Verification items for the finished model (mm, model axes). A direction names the side the tool comes from. Coordinates: 2 decimals unless noted, no trailing zeros. Write each loop counter-clockwise with the first axis right and the second up, starting at its lowest first coordinate (ties: lowest second). Pieces come first, ordered by that corner, then holes. Notation, with made-up numbers: M 72.25,24.5 L 126.25,24.5 A15 cw 126.25,40.5 Z; hole C -17,-39 d6. An arc over 180 degrees is marked long. One line per item, written item: value.
```python
from build123d import *

# Parameters (mm, degrees)
ESQUISSE1_R        = 20
ESQUISSE1_R_2      = 15
ESQUISSE1_R_3      = 6
BOSS_EXTRU_1_DEPTH = 1
ESQUISSE1_3_R      = 15
ESQUISSE1_3_R_2    = 6
BOSS_EXTRU_2_DEPTH = 12
ESQUISSE2_R        = 20
ESQUISSE2_R_2      = 15
ESQUISSE2_R_3      = 6
BOSS_EXTRU_4_DEPTH = 1


with BuildPart() as part:
    # Esquisse1 → Boss.-Extru.1 (new body)
    with BuildSketch(Plane(origin=(0, 0, 0), x_dir=(1, 0, 0), z_dir=(0, 1, 0))):
        with Locations(Location((0, 0, 0), (0, 0, 270))):
            Circle(ESQUISSE1_R)
        Circle(ESQUISSE1_R_2, mode=Mode.SUBTRACT)
        Circle(ESQUISSE1_R_2)
        with Locations(Location((0, 0, 0), (0, 0, 270))):
            Circle(ESQUISSE1_R_3, mode=Mode.SUBTRACT)
    extrude(amount=-BOSS_EXTRU_1_DEPTH)

    # Esquisse1_3 → Boss.-Extru.2 (add)
    with BuildSketch(Plane(origin=(0, 0, 0), x_dir=(1, 0, 0), z_dir=(0, 1, 0))):
        with Locations(Location((0, 0, 0), (0, 0, 270))):
            Circle(ESQUISSE1_3_R)
        with Locations(Location((0, 0, 0), (0, 0, 270))):
            Circle(ESQUISSE1_3_R_2, mode=Mode.SUBTRACT)
    extrude(amount=BOSS_EXTRU_2_DEPTH)

    # Esquisse2 → Boss.-Extru.4 (add)
    with BuildSketch(Plane(origin=(0, 12, 0), x_dir=(1, 0, 0), z_dir=(0, 1, 0))):
        with Locations(Location((0, 0, 0), (0, 0, 270))):
            Circle(ESQUISSE2_R)
        with Locations(Location((0, 0, 0), (0, 0, 270))):
            Circle(ESQUISSE2_R_2, mode=Mode.SUBTRACT)
        with Locations(Location((0, 0, 0), (0, 0, 270))):
            Circle(ESQUISSE2_R_2)
        with Locations(Location((0, 0, 0), (0, 0, 270))):
            Circle(ESQUISSE2_R_3, mode=Mode.SUBTRACT)
    extrude(amount=BOSS_EXTRU_4_DEPTH)


solid = part.part
```
Item 1: Draft check along Y on faces 3 (the face through (0.66, 5.916, -14.985)), 4 (the face through (5, -1, 4)), 5 (the face through (-19.524, -0.493, -4.336)). Enter one of: released by +Y, released by -Y, zero draft, split by the parting line, or undercut.
The answers:
face 3: undercut
face 4: released by -Y
face 5: zero draft
Item 2: Cross-section at D-D, the plane x = 7. Enter the section's corners in (y, z) (1 decimal), and give its area (3 significant figures).
The answers:
outline: M -1,-18.7 L 0,-18.7 L 0,-13.3 L 12,-13.3 L 12,-18.7 L 13,-18.7 L 13,18.7 L 12,18.7 L 12,13.3 L 0,13.3 L 0,18.7 L -1,18.7 Z
area: 393 mm²
Item 3: Access from +Z, -Z, +X, -X, +Y, -Y to the whole of each face (thin tool, end or side, straight path). Record for faces 1 (the face through (5, 13, 4)), 2 (the face through (15, 12, 3)).
The answers:
face 1: +Z, -Z, +X, -X, +Y
face 2: none
Item 4: Cross-section at B-B, the plane x = 0. Enter the section's corners in (y, z).
The answers:
outline: M -1,-20 L 0,-20 L 0,-15 L 12,-15 L 12,-20 L 13,-20 L 13,-6 L -1,-6 Z; M -1,6 L 13,6 L 13,20 L 12,20 L 12,15 L 0,15 L 0,20 L -1,20 Z
Item 5: Scan lines: line 1 (Y direction, x = -14, z = -13); line 2 (X direction, y = 8.5, z = 0); line 3 (Z direction, x = -1, y = 10.75). Record each from-to range of solid material in increasing order.
The answers:
line 1: y = -1 to 0, 12 to 13
line 2: x = -15 to -6, 6 to 15
line 3: z = -14.97 to -5.92, 5.92 to 14.97
Item 6: Cross-section at A-A, the plane z = 0. Enter the section's corners in (x, y).
The answers:
outline: M -20,-1 L -6,-1 L -6,13 L -20,13 L -20,12 L -15,12 L -15,0 L -20,0 Z; M 6,-1 L 20,-1 L 20,0 L 15,0 L 15,12 L 20,12 L 20,13 L 6,13 Z
Item 7: Go/stop test with flat-tipped pins: P1, Ø2, axis at x = 8.5, y = 3, coming from the +Z side; P2, Ø1.5, axis at y = 7.5, z = -4.5, coming from the -X side; P3, Ø2, axis at x = 12.5, y = 7.5, coming from the -Z side. Record where each tip stops, or that it passes through.
The answers:
P1: stops at z = 12.99
P2: stops at x = -14.52
P3: stops at z = -9.63
Item 8: Cross-section at C-C, the plane y = 2.25. Enter the section's corners in (x, z).
The answers:
outline: C 0,0 d30; hole C 0,0 d12
